Design review of the part built by this model. Coordinates are the model's own, in mm. A direction names the side the tool comes from. Give positions to 0.01 mm unless a question says otherwise; leave off trailing zeros. Return JSON: item names as keys, results as strings. Group by question number.
from build123d import *

# Parameters (mm, degrees)
SKETCH1_R                  = 2.6
SKETCH1_W                  = 70
SKETCH1_H                  = 10.2
SKETCH1_W_2                = 70.1
SKETCH1_H_2                = 10.3
SKETCH1_W_3                = 70.2
SKETCH1_H_3                = 10.4
SKETCH1_W_4                = 70.3
SKETCH1_H_4                = 10.5
SKETCH1_W_5                = 70.4
SKETCH1_H_5                = 10.6
BOSS_EXTRUDE1_DEPTH        = 9.5
F_3_3_3_3_DIAMETER_HOLE1_D = 3.3
F_3_0_3_DIAMETER_HOLE1_D   = 3


with BuildPart() as part:
    # Sketch1 → Boss-Extrude1 (new body)
    with BuildSketch(Plane.XY):
        Polygon((-250, -25), (-259.5, -25), (-259.5, 25), (-250, 25), (-250, 50), (250, 50), (250, 25), (259.5, 25), (259.5, -25), (250, -25), (250, -50), (-250, -50), align=None)
        with Locations((-233, -42)):
            Circle(SKETCH1_R, mode=Mode.SUBTRACT)
        with Locations((-197, -42)):
            Circle(SKETCH1_R, mode=Mode.SUBTRACT)
        with Locations((-197, -8)):
            Circle(SKETCH1_R, mode=Mode.SUBTRACT)
        with Locations((-233, -8)):
            Circle(SKETCH1_R, mode=Mode.SUBTRACT)
        with Locations((-197, 42)):
            Circle(SKETCH1_R, mode=Mode.SUBTRACT)
        with Locations((-197, 8)):
            Circle(SKETCH1_R, mode=Mode.SUBTRACT)
        with Locations((-233, 8)):
            Circle(SKETCH1_R, mode=Mode.SUBTRACT)
        with Locations((-233, 42)):
            Circle(SKETCH1_R, mode=Mode.SUBTRACT)
        with Locations((233, 42)):
            Circle(SKETCH1_R, mode=Mode.SUBTRACT)
        with Locations((233, 8)):
            Circle(SKETCH1_R, mode=Mode.SUBTRACT)
        with Locations((197, 8)):
            Circle(SKETCH1_R, mode=Mode.SUBTRACT)
        with Locations((197, 42)):
            Circle(SKETCH1_R, mode=Mode.SUBTRACT)
        with Locations((233, -8)):
            Circle(SKETCH1_R, mode=Mode.SUBTRACT)
        with Locations((197, -8)):
            Circle(SKETCH1_R, mode=Mode.SUBTRACT)
        with Locations((197, -42)):
            Circle(SKETCH1_R, mode=Mode.SUBTRACT)
        with Locations((233, -42)):
            Circle(SKETCH1_R, mode=Mode.SUBTRACT)
        with Locations((-17.5, -37)):
            Circle(SKETCH1_R, mode=Mode.SUBTRACT)
        with Locations((17.5, -37)):
            Circle(SKETCH1_R, mode=Mode.SUBTRACT)
        with Locations((17.5, -13)):
            Circle(SKETCH1_R, mode=Mode.SUBTRACT)
        with Locations((-17.5, -13)):
            Circle(SKETCH1_R, mode=Mode.SUBTRACT)
        with Locations((-135, 24.9)):
            Rectangle(SKETCH1_W, SKETCH1_H, mode=Mode.SUBTRACT)
        with Locations((-134.95, -24.85)):
            Rectangle(SKETCH1_W_2, SKETCH1_H_2, mode=Mode.SUBTRACT)
        with Locations((0, 24.8)):
            Rectangle(SKETCH1_W_3, SKETCH1_H_3, mode=Mode.SUBTRACT)
        with Locations((134.85, 24.75)):
            Rectangle(SKETCH1_W_4, SKETCH1_H_4, mode=Mode.SUBTRACT)
        with Locations((134.8, -24.7)):
            Rectangle(SKETCH1_W_5, SKETCH1_H_5, mode=Mode.SUBTRACT)
    extrude(amount=BOSS_EXTRUDE1_DEPTH)

    # Ø3.3 (3.3) Diameter Hole1 (through all)
    with Locations(Plane.XY.offset(9.5)):
        with Locations((-235.3, 25), (-218, 25), (-218, -25), (-235.3, -25), (235.3, -25), (218, -25), (218, 25), (235.3, 25)):
            Hole(F_3_3_3_3_DIAMETER_HOLE1_D / 2)

    # Ø3.0 (3) Diameter Hole1 (through all)
    with Locations(Plane.XY.offset(9.5)):
        with Locations((-250, 26.5), (-250, -26.5), (-168.5, 30), (-101.5, 30), (-101.5, 19.8), (-168.5, 19.8), (-168.5, -19.7), (-168.5, -30), (-101.4, -19.7), (-101.4, -30), (-33.6, 30), (-33.6, 19.6), (33.6, 30), (33.6, 19.6), (168.5, 30), (168.5, 19.5), (101.2, 30), (101.2, 19.5), (101.1, -19.4), (101.1, -30), (168.5, -19.4), (168.5, -30), (250, 26.5), (250, -26.5)):
            Hole(F_3_0_3_DIAMETER_HOLE1_D / 2)


solid = part.part
Q1. Take a section at A-A, the plane z = 3. Count the separate pieces of the cut face and the enclosed holes in it, plus the area to 3 significant figures.
Q2. Insertion check: pin 1 (3 mm diameter, centred on x = -252.5, z = 6.5, fed in from -Y). The pin has a flat end and moves straight along its axis. Give the tip position at first contact, or say it passes through.
Q3. For L1, parallel to Y at x = -121, z = 2.5; L2, parallel to Y at x = -197, z = 6.75; L3, parallel to Y at x = 218, z = 5.5, list the stretches that pass through material, from the lowest coordinate up. Write a range as from..to.
Q4. Tool access review of faces 1 (the face through (99.6, -25, 5)), 2 (the face through (-255, 25, 5)), 3 (the face through (-3, 50, 5)): name each direction out of +Z, -Z, +X, -X, +Y, -Y from which nothing blocks a thin tool from reaching the whole face with its end or side.
Q5. Mouldability with a two-part tool opening along Y and no side actions: class faces 4 (the face through (-259.5, 0, 5)), 5 (the face through (-255, -25, 5)), 6 (the face through (0, 30, 5)) as +Y half, -Y half, draft (parallel to the pull), parting line (faces both ways), or undercut.
Final values:
{
 "1": {"separate pieces": "1", "enclosed holes": "33", "area": "46,700 mm²"},
 "2": {"pin 1": "stops at y = -25"},
 "3": {"L1": "y = -50..-30, -19.7..19.8, 30..50", "L2": "y = -50..-44.6, -39.4..-10.6, -5.4..5.4, 10.6..39.4, 44.6..50", "L3": "y = -50..-26.65, -23.35..23.35, 26.65..50"},
 "4": {"face 1": "+Z, -Z", "face 2": "+Z, -Z, -X, +Y", "face 3": "+Z, -Z, +X, -X, +Y"},
 "5": {"face 4": "draft", "face 5": "-Y half", "face 6": "undercut"}
}
